```python
from build123d import *

# Parameters (mm, degrees)
SKETCH_W                   = 74
SKETCH_H                   = 74
PAD_DEPTH                  = 3
SKETCH002_W                = 64
SKETCH002_H                = 64
SKETCH002_W_2              = 60
SKETCH002_H_2              = 60
PAD001_DEPTH               = 35
SKETCH003_R                = 1.5
POCKET_DEPTH               = 225.675651
PAD002_DEPTH               = 32
SKETCH005_R                = 2.4
POCKET001_DEPTH            = 10
SKETCH003_MIRRORED_2_R     = 1.5
POCKET_MIRRORED_2_DEPTH    = 225.675651
PAD002_MIRRORED_2_DEPTH    = 32
SKETCH005_MIRRORED_2_R     = 2.4
POCKET001_MIRRORED_2_DEPTH = 10


with BuildPart() as part:
    # Sketch → Pad (new body)
    with BuildSketch(Plane.XY):
        Rectangle(SKETCH_W, SKETCH_H)
    extrude(amount=PAD_DEPTH)

    # Sketch002 (on Face5 of Pad) → Pad001 (join)
    with BuildSketch(Plane(origin=(0, 0, 0), x_dir=(1, 0, 0), z_dir=(0, 0, -1))):
        Rectangle(SKETCH002_W, SKETCH002_H)
        Rectangle(SKETCH002_W_2, SKETCH002_H_2, mode=Mode.SUBTRACT)
    extrude(amount=PAD001_DEPTH)

    # Sketch003 (on Face4 of Pad001) → Pocket (cut, through all)
    with BuildSketch(Plane(origin=(0, 0, 0), x_dir=(1, 0, 0), z_dir=(0, 0, -1))):
        with Locations((-34, 34)):
            Circle(SKETCH003_R)
    pocket = extrude(amount=-POCKET_DEPTH, mode=Mode.SUBTRACT)

    # Sketch004 (on Face17 of Pocket) → Pad002 (join)
    with BuildSketch(Plane(origin=(0, 0, 0), x_dir=(1, 0, 0), z_dir=(0, 0, -1))):
        with BuildLine():
            ThreePointArc((-30, 22), (-24.343146, 24.343146), (-22, 30))
            Line((-30, 30), (-22, 30))
            Line((-30, 30), (-30, 22))
        make_face()
    pad002 = extrude(amount=PAD002_DEPTH)

    # Sketch005 (on Face17 of Pad002) → Pocket001 (cut)
    with BuildSketch(Plane(origin=(0, 0, -32), x_dir=(1, 0, 0), z_dir=(0, 0, -1))):
        with Locations((-27, 27)):
            Circle(SKETCH005_R)
    pocket001 = extrude(amount=-POCKET001_DEPTH, mode=Mode.SUBTRACT)

    # Sketch003 Mirrored 2 → Pocket Mirrored 2 (cut, through all)
    with BuildSketch(Plane(origin=(0, 0, 0), x_dir=(-1, 0, 0), z_dir=(0, 0, 1))):
        with Locations((-34, 34)):
            Circle(SKETCH003_MIRRORED_2_R)
    pocket_mirrored_2 = extrude(amount=POCKET_MIRRORED_2_DEPTH, mode=Mode.SUBTRACT)

    # Sketch004 Mirrored 2 → Pad002 Mirrored 2 (add)
    with BuildSketch(Plane(origin=(0, 0, 0), x_dir=(-1, 0, 0), z_dir=(0, 0, 1))):
        with BuildLine():
            ThreePointArc((-30, 22), (-24.343146, 24.343146), (-22, 30))
            Line((-30, 30), (-22, 30))
            Line((-30, 30), (-30, 22))
        make_face()
    pad002_mirrored_2 = extrude(amount=-PAD002_MIRRORED_2_DEPTH)

    # Sketch005 Mirrored 2 → Pocket001 Mirrored 2 (cut)
    with BuildSketch(Plane(origin=(0, 0, -32), x_dir=(-1, 0, 0), z_dir=(0, 0, 1))):
        with Locations((-27, 27)):
            Circle(SKETCH005_MIRRORED_2_R)
    pocket001_mirrored_2 = extrude(amount=POCKET001_MIRRORED_2_DEPTH, mode=Mode.SUBTRACT)

    # Mirrored001: Pocket, Pad002, Pocket001, Pocket Mirrored 2, Pad002 Mirrored 2, Pocket001 Mirrored 2 across Sketch003 H_Axis
    add(pocket.mirror(Plane(origin=(0, 0, 0), x_dir=(0, 0, -1), z_dir=(0, -1, 0))), mode=Mode.SUBTRACT)
    add(pad002.mirror(Plane(origin=(0, 0, 0), x_dir=(0, 0, -1), z_dir=(0, -1, 0))))
    add(pocket001.mirror(Plane(origin=(0, 0, 0), x_dir=(0, 0, -1), z_dir=(0, -1, 0))), mode=Mode.SUBTRACT)
    add(pocket_mirrored_2.mirror(Plane(origin=(0, 0, 0), x_dir=(0, 0, -1), z_dir=(0, -1, 0))), mode=Mode.SUBTRACT)
    add(pad002_mirrored_2.mirror(Plane(origin=(0, 0, 0), x_dir=(0, 0, -1), z_dir=(0, -1, 0))))
    add(pocket001_mirrored_2.mirror(Plane(origin=(0, 0, 0), x_dir=(0, 0, -1), z_dir=(0, -1, 0))), mode=Mode.SUBTRACT)


solid = part.part
```
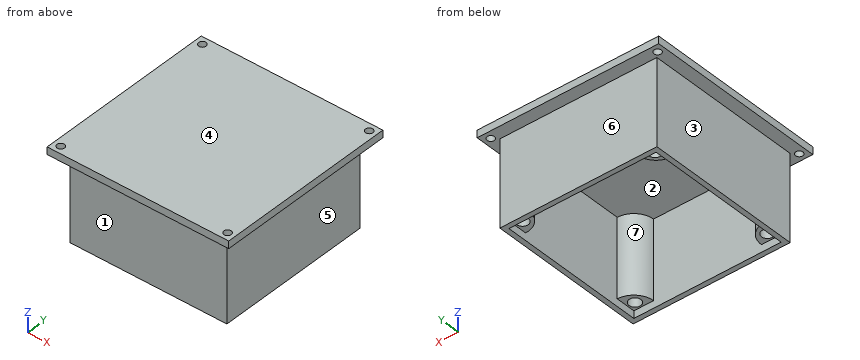
Build history of the part. All positions in model axes, mm. Face numbers are marked on the shaded views. A direction names the side the tool comes from. Round coordinates to 2 decimals unless told otherwise and drop trailing zeros. Loops run counter-clockwise (first coordinate to the right, second up) from the corner with the lowest first, then second, coordinate; pieces in that order, holes last.
Item 1: Which spindle directions (+Z, -Z, +X, -X, +Y, -Y) get a long thin tool onto all of the face, cutting with end or side? Do the marked faces 1, 2, 3 and 4. Say none if no direction does.
Item 2: Saw through at A-A (y = -34). List the corners of the cut face in (x, z), then the cut area to 3 significant figures.
Item 3: Two-plate mould, pull along Y, no slides. Class the marked faces 5, 6 and 7: released by +Y, released by -Y, zero draft, split by the parting line, or undercut.
Item 4: Pin check, flat tips, straight feed: P1, Ø10, axis at y = 24, z = -20.5, coming from the -X side; P2, Ø8, axis at x = 22.5, y = -5.5, coming from the -Z side; P3, Ø1, axis at y = -27.5, z = -9.5, coming from the +X side; P4, Ø7.5, axis at x = -27, y = -27, coming from the -Z side. Stop position of each tip, or through.
Item 5: Saw through at C-C (x = -9). List the corners of the cut face in (y, z).
Item 6: Drill centre lines: line 1 along Y through (x, z) = (34, 1); line 2 along Y through (x, z) = (27, -25). Where is each one in solid material? Low to high.
Item 7: Saw through at B-B (z = -6). List the corners of the cut face in (x, y).
Worked answers:
1. face 1: -Z, +X, -X, -Y
1. face 2: -Z
1. face 3: -Z, -X, +Y, -Y
1. face 4: +Z, +X, -X, +Y, -Y
2. outline: (-37, 0) - (-35.5, 0) - (-35.5, 3) - (-37, 3) - close; (-32.5, 0) - (32.5, 0) - (32.5, 3) - (-32.5, 3) - close; (35.5, 0) - (37, 0) - (37, 3) - (35.5, 3) - close
2. area: 204 mm2
3. face 5: zero draft
3. face 6: released by +Y
3. face 7: undercut
4. P1: stops at x = -32
4. P2: stops at z = 0
4. P3: stops at x = 32
4. P4: stops at z = -35
5. outline: (-37, 0) - (-32, 0) - (-32, -35) - (-30, -35) - (-30, 0) - (30, 0) - (30, -35) - (32, -35) - (32, 0) - (37, 0) - (37, 3) - (-37, 3) - close
6. line 1: y = -37 to -35.5, -32.5 to 32.5, 35.5 to 37
6. line 2: y = -32 to -29.4, -24.6 to -22.58, 22.58 to 24.6, 29.4 to 32
7. outline: (-32, -32) - (32, -32) - (32, 32) - (-32, 32) - close; hole (-30, -22) arc R8 cw to (-22, -30) - (22, -30) arc R8 cw to (30, -22) - (30, 22) arc R8 cw to (22, 30) - (-22, 30) arc R8 cw to (-30, 22) - close
